Geometry check sheet. Reference: the model listing, model coordinates, mm. Give positions to 0.01 mm unless a question says otherwise; leave off trailing zeros. Write each loop counter-clockwise with the first axis right and the second up, starting at its lowest first coordinate (ties: lowest second). Pieces come first, ordered by that corner, then holes. Notation, with made-up numbers: (78, -12) - (130, -12) arc R28 cw to (130, 10) - close; hole circle Ø5 at (-4.75, -18). An arc over 180 degrees is marked (long way). One line per question, with ' | ' between items. Start each with the question number.
Q1. Thickness scan on L1, parallel to Y at x = -46.89, z = 2; L2, parallel to X at y = -9, z = 2.65; L3, parallel to X at y = -4, z = 1.3. Record the ranges inside material, lowest first. Write a range as [from, to].
Q2. Gauge pin test, flat ends, axial feed: P1, Ø10, axis at x = -110, y = 0, coming from the +Z side; P2, Ø0.9, axis at x = -59, z = 2, coming from the +Y side; P3, Ø1.5, axis at y = -5, z = 0.5, coming from the +X side. Record the tip position at first contact, or that the pin passes through.
Q3. Section check D-D on y = -17.25. Record the boundary of the cut face in (x, z).
Q4. Section check C-C on z = 1.6. Count the separate pieces of the cut face and the enclosed holes in it, and give its area (3 significant figures).
Q5. Section check A-A on y = 0. Record the boundary of the cut face in (x, z), and give its area (3 significant figures).
Q6. Section check B-B on x = -46.89. Record the boundary of the cut face in (y, z), and give its area (3 significant figures).
```python
from build123d import *

# Parameters (mm, degrees)
ESQUISSE1_R        = 5.5
ESQUISSE1_R_2      = 1.75
ESQUISSE1_R_3      = 2.1
BOSS_EXTRU_1_DEPTH = 3


with BuildPart() as part:
    # Esquisse1 → Boss.-Extru.1 (new body)
    with BuildSketch(Plane.XY):
        with BuildLine():
            Line((-110, 8.5), (-19.20286437, 8.5))
            ThreePointArc((-19.20286437, 8.5), (21, 0), (-19.20286437, -8.5))
            Line((-19.20286437, -8.5), (-110, -8.5))
            ThreePointArc((-110, -8.5), (-118.5, 0), (-110, 8.5))
        make_face()
        with Locations((-110, 0)):
            Circle(ESQUISSE1_R, mode=Mode.SUBTRACT)
        Circle(ESQUISSE1_R, mode=Mode.SUBTRACT)
        with Locations((0, 17.25)):
            Circle(ESQUISSE1_R_2, mode=Mode.SUBTRACT)
        with Locations((17.25, 0)):
            Circle(ESQUISSE1_R_2, mode=Mode.SUBTRACT)
        with Locations((0, -17.25)):
            Circle(ESQUISSE1_R_2, mode=Mode.SUBTRACT)
        with Locations((-17.25, 0)):
            Circle(ESQUISSE1_R_2, mode=Mode.SUBTRACT)
        with Locations((-75.14, 0)):
            Circle(ESQUISSE1_R_3, mode=Mode.SUBTRACT)
        with Locations((-46.89, 0)):
            Circle(ESQUISSE1_R_3, mode=Mode.SUBTRACT)
    extrude(amount=BOSS_EXTRU_1_DEPTH)


solid = part.part
```
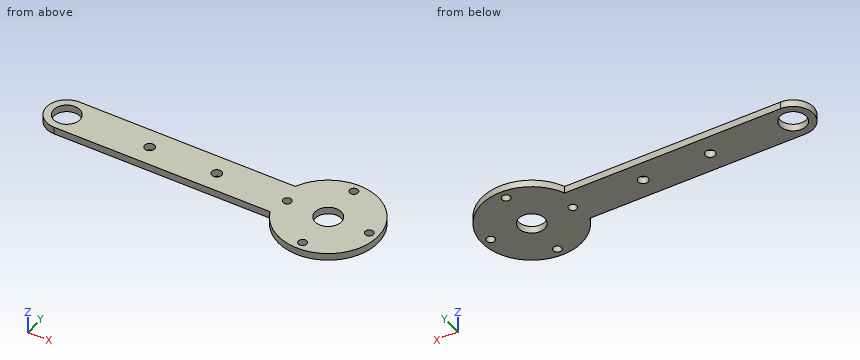
Working result:
1) L1: y = [-8.5, -2.1], [2.1, 8.5] | L2: x = [-18.97, 18.97] | L3: x = [-117.5, -113.77], [-106.23, -3.77], [3.77, 20.62]
2) P1: passes through | P2: stops at y = 8.5 | P3: stops at x = 20.57
3) outline: (-11.98, 0) - (-1.75, 0) - (-1.75, 3) - (-11.98, 3) - close; (1.75, 0) - (11.98, 0) - (11.98, 3) - (1.75, 3) - close
4) separate pieces: 1 | enclosed holes: 8 | area: 2,770 mm2
5) outline: (-118.5, 0) - (-115.5, 0) - (-115.5, 3) - (-118.5, 3) - close; (-104.5, 0) - (-77.24, 0) - (-77.24, 3) - (-104.5, 3) - close; (-73.04, 0) - (-48.99, 0) - (-48.99, 3) - (-73.04, 3) - close; (-44.79, 0) - (-19, 0) - (-19, 3) - (-44.79, 3) - close; (-15.5, 0) - (-5.5, 0) - (-5.5, 3) - (-15.5, 3) - close; (5.5, 0) - (15.5, 0) - (15.5, 3) - (5.5, 3) - close; (19, 0) - (21, 0) - (21, 3) - (19, 3) - close | area: 306 mm2
6) outline: (-8.5, 0) - (-2.1, 0) - (-2.1, 3) - (-8.5, 3) - close; (2.1, 0) - (8.5, 0) - (8.5, 3) - (2.1, 3) - close | area: 38.4 mm2
